The model under review builds one solid part; all positions refer to its coordinate system, in mm. A direction names the side the tool comes from. Coordinates: 2 decimals unless noted, no trailing zeros. Loops run counter-clockwise (first coordinate to the right, second up) from the corner with the lowest first, then second, coordinate; pieces in that order, holes last. Notation, with made-up numbers: M 54.25,85.25 L 111.25,85.25 A4 cw 111.25,89.25 Z; hole C 4.5,56 d1. An arc over 180 degrees is marked long. Use one line per item in the form item = value.
```python
from build123d import *

# Parameters (mm, degrees)
SKETCH2_R           = 14.306408623
BOSS_EXTRUDE1_DEPTH = 10
SKETCH3_W           = 28.579032966
SKETCH3_H           = 1.390030786
BOSS_EXTRUDE2_DEPTH = 45
SKETCH4_W           = 6
SKETCH4_H           = 6
BOSS_EXTRUDE3_DEPTH = 6


with BuildPart() as part:
    # Sketch1 → Revolve1 (revolve)
    with BuildSketch(Plane(origin=(0, 0, 0), x_dir=(1, 0, 0), z_dir=(0, 1, 0))):
        with BuildLine():
            Line((19.306408623, 0), (0, 0))
            Line((0, 0), (0, 19.306408623))
            ThreePointArc((0, 19.306408623), (13.651692458, 13.651692458), (19.306408623, 0))
        make_face()
    revolve(axis=Axis((0, 0, 0), (0, 0, -1)))

    # Sketch2 → Boss-Extrude1 (add)
    with BuildSketch(Plane.XY):
        Circle(SKETCH2_R)
    extrude(amount=BOSS_EXTRUDE1_DEPTH)

    # Sketch3 → Boss-Extrude2 (add)
    with BuildSketch(Plane.XY.offset(10)):
        Rectangle(SKETCH3_W, SKETCH3_H)
    extrude(amount=BOSS_EXTRUDE2_DEPTH)

    # Sketch4 → Boss-Extrude3 (add)
    with BuildSketch(Plane(origin=(0, 0.695015393, 0), x_dir=(1, 0, 0), z_dir=(0, 1, 0))):
        with Locations((7, -53)):
            Rectangle(SKETCH4_W, SKETCH4_H)
        with Locations((0, -53)):
            Rectangle(SKETCH4_W, SKETCH4_H)
        with Locations((-7, -53)):
            Rectangle(SKETCH4_W, SKETCH4_H)
    extrude(amount=BOSS_EXTRUDE3_DEPTH)


solid = part.part
```
1. Add section A-A (x = 0). State the section outline as (y, z) points, then the cut area to 3 significant figures.
Response values:
outline = M -19.31,0 A19.31 ccw 19.31,0 L 14.31,0 L 14.31,10 L 0.7,10 L 0.7,50 L 6.7,50 L 6.7,56 L 0.7,56 L 0.7,55 L -0.7,55 L -0.7,10 L -14.31,10 L -14.31,0 Z
area = 970 mm^2
2. Add section D-D (y = -11.5). State the section outline as (x, z) points, then the cut area to 3 significant figures.
Response values:
outline = M -15.51,0 A15.51 ccw 15.51,0 L 8.51,0 L 8.51,10 L -8.51,10 L -8.51,0 Z
area = 548 mm^2
3. Insertion check: P1, Ø1.5, axis at x = 6, z = -4, coming from the +Y side; P2, Ø3, axis at x = 7.5, z = 53.5, coming from the +Y side (3 decimals); P3, Ø2, axis at y = 8.5, z = -7.5, coming from the +X side. Each pin has a flat end and moves straight along its axis. Give the tip position at first contact, or say it passes through.
Response values:
P1 = 18.19
P2 = 6.695
P3 = 16.31
4. The part is to be moulded in two halves that separate along X. For faces 4 (the face through (-3.101, -13.966, 4.93)), 5 (the face through (4, 4, 53)), 6 (the face through (10, 4, 53)), 7 (the face through (0, -6, 10)), say which applies: pulls with the +X half, pulls with the -X half, needs draft (parallel to the pull), parting line crosses it, or undercut.
Response values:
face_4 = parting line crosses it
face_5 = undercut
face_6 = pulls with the +X half
face_7 = needs draft
5. Machinability: for faces 1 (the face through (0, 4, 50)), 2 (the face through (0, 6.695, 53)), 3 (the face through (3, 4, 53)), which of the approach directions +Z, -Z, +X, -X, +Y, -Y give a long, thin tool a straight path to every point of the face, cutting with its end or side? Answer none if there is none.
Response values:
face_1 = +X, -X, +Y
face_2 = +Z, +X, -X, +Y
face_3 = +Z, +Y
6. Add section C-C (x = -13.5). State the section outline as (y, z) points.
Response values:
outline = M -13.8,0 A13.8 ccw 13.8,0 L 4.74,0 L 4.74,10 L 0.7,10 L 0.7,55 L -0.7,55 L -0.7,10 L -4.74,10 L -4.74,0 Z
7. Wall thickness on line 1 along Z through (x, y) = (5, -12); line 2 along Y through (x, z) = (-11.5, 31.5); line 3 along X through (y, z) = (-1, 5): over which ranges is each line inside the solid? List them lowest first. Write a range as from..to.
Response values:
line_1 = -14.27..10
line_2 = -0.7..0.7
line_3 = -14.27..14.27
8. Add section B-B (y = -5.5). State the section outline as (x, z) points, then the cut area to 3 significant figures.
Response values:
outline = M -18.51,0 A18.51 ccw 18.51,0 L 13.21,0 L 13.21,10 L -13.21,10 L -13.21,0 Z
area = 802 mm^2
